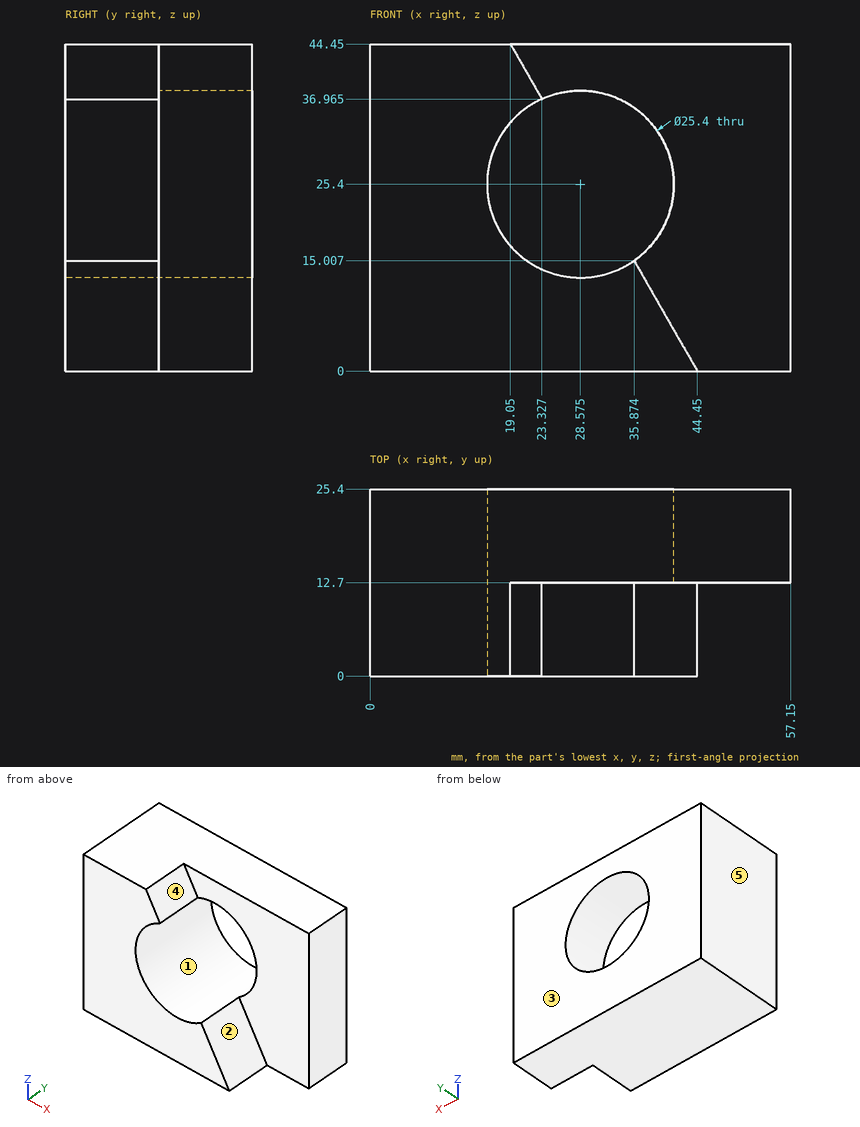
Study the drawing (mm; zero at the part's minimum x, y, z) and answer. A direction names the side the tool comes from. Coordinates: 2 decimals unless noted, no trailing zeros. Answer in a Markdown table with one row per item. Add a question column.
Item 1: Each of these flat-tipped pins is pushed along its axis until it touches: P1, Ø10, axis at x = 25.5, z = 17.5, coming from the +Y side; P2, Ø1.5, axis at y = 4.5, z = 25.5, coming from the +X side. Where does it stop, or does it pass through?
Item 2: Find the intervals of material crossed by L1, parallel to X at y = 12.25, z = 25.4 (1 decimal); L2, parallel to Y at x = 36.5, z = 38.5; L3, parallel to Z at x = 20, y = 23.75, in increasing order. Write a range as from..to.
Item 3: Determine the mould class of the marked faces 1, 2 and 3 for opening direction X: +X half, -X half, draft (parallel to the pull), parting line (faces both ways), or undercut.
Item 4: Which of the six approach directions +Z, -Z, +X, -X, +Y, -Y give full straight-line access (tool end or side, diameter ignored) to the marked faces 4 and 5?
Result set:
| question | item | result |
|---|---|---|
| 1 | P1 | stops at y = 25.4 |
| 1 | P2 | stops at x = 15.9 |
| 2 | L1 | x = 0..15.9 |
| 2 | L2 | y = 12.7..25.4 |
| 2 | L3 | z = 0..16.03, 34.77..44.45 |
| 3 | face 1 | undercut |
| 3 | face 2 | +X half |
| 3 | face 3 | draft |
| 4 | face 4 | +Z, +X, -Y |
| 4 | face 5 | +Z, -Z, -X, +Y, -Y |
